Design review of the part shown in the three views and the two pictorial views. Dimensions are in mm from the part's minimum x, y and z. A direction names the side the tool comes from. Coordinates: 2 decimals unless noted, no trailing zeros. Loops run counter-clockwise (first coordinate to the right, second up) from the corner with the lowest first, then second, coordinate; pieces in that order, holes last. Notation, with made-up numbers: (7, 26) - (48, 26) arc R19 cw to (48, 46) - close; hole circle Ø1 at (-33, 14.25). An arc over 180 degrees is marked (long way). One line per item, written item: value. Start each with the question number.
1. To check wall thickness, follow line 1 (Z direction, x = 21, y = 15); line 2 (Z direction, x = 26, y = 7); line 3 (Y direction, x = 14, z = 54). State the ranges of each line that lie inside material, in increasing order. Write a range as from..to.
2. For the marked faces 1 and 2, list the 3-axis set-ups (+Z, -Z, +X, -X, +Y, -Y) from which the entire face can be reached by the end or side of a thin tool; tool diameter is ignored.
3. Take a section at D-D, the plane z = 22.5. State the section outline as (x, y) points.
4. Insertion check: pin 1 (8 mm diameter, centred on y = 23.5, z = 45, fed in from +X); pin 2 (3 mm diameter, centred on x = 23.5, y = 30, fed in from +Z). Each pin has a flat end and moves straight along its axis. Give the tip position at first contact, or say it passes through.
5. Take a section at A-A, the plane x = 17.5. State the section outline as (y, z) points, and give its area (3 significant figures).
6. Take a section at C-C, the plane x = 22.5. State the section outline as (y, z) points.
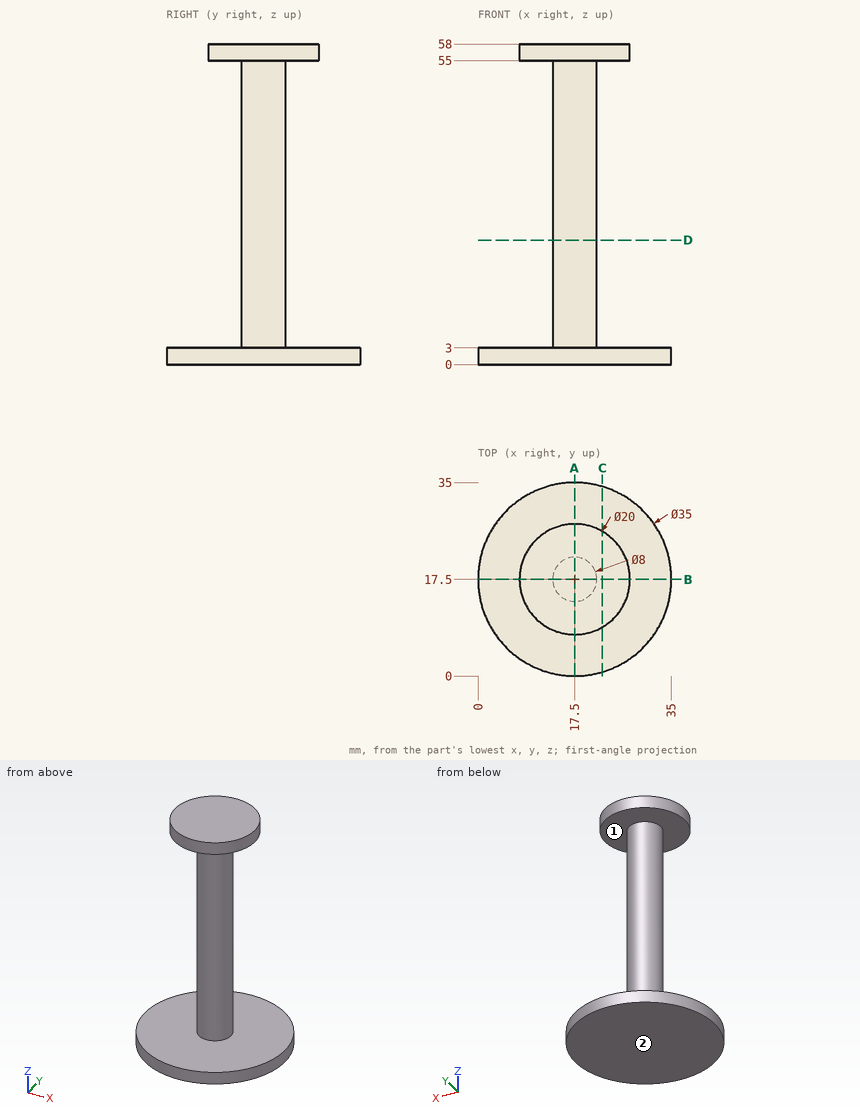
Solutions:
1. line 1: 0..3, 55..58
1. line 2: 0..3
1. line 3: 15.56..19.44
2. face 1: none
2. face 2: -Z, +X, -X, +Y, -Y
3. outline: circle Ø8 at (17.5, 17.5)
4. pin 1: x = 20.96
4. pin 2: z = 3
5. outline: (0, 0) - (35, 0) - (35, 3) - (21.5, 3) - (21.5, 55) - (27.5, 55) - (27.5, 58) - (7.5, 58) - (7.5, 55) - (13.5, 55) - (13.5, 3) - (0, 3) - close
5. area: 581 mm2
6. outline: (0.73, 0) - (34.27, 0) - (34.27, 3) - (0.73, 3) - close; (8.84, 55) - (26.16, 55) - (26.16, 58) - (8.84, 58) - close
